from build123d import *

# Parameters (mm, degrees)
SKETCH1_R           = 102.5
BOSS_EXTRUDE1_DEPTH = 41
BOSS_EXTRUDE2_START = 41
SKETCH1_3_R         = 102.5
BOSS_EXTRUDE2_DEPTH = 191
BOSS_EXTRUDE3_START = 232
SKETCH1_4_R         = 102.5
BOSS_EXTRUDE3_DEPTH = 41
SKETCH3_R           = 27.5
SKETCH3_R_2         = 23
SKETCH3_R_3         = 5
BOSS_EXTRUDE4_DEPTH = 10
SKETCH3_3_R         = 23
SKETCH3_3_R_2       = 27.5
BOSS_EXTRUDE5_DEPTH = 273


with BuildPart() as part:
    # Sketch1 → Boss-Extrude1 (new body)
    with BuildSketch(Plane.XY):
        with BuildLine():
            Line((120, 77.892348876), (120, 0))
            Line((120, 0), (80, 0))
            Line((80, 0), (80, 42.168378274))
            ThreePointArc((80, 42.168378274), (0, 19.5), (-80, 42.168378274))
            Line((-80, 42.168378274), (-80, 0))
            Line((-80, 0), (-120, 0))
            Line((-120, 0), (-120, 77.892348876))
            ThreePointArc((-120, 77.892348876), (0, 324.5), (120, 77.892348876))
        make_face()
        with Locations((0, 172)):
            Circle(SKETCH1_R, mode=Mode.SUBTRACT)
        with Locations((0, 172)):
            Circle(SKETCH1_R)
    extrude(amount=BOSS_EXTRUDE1_DEPTH)

    # Sketch1<3> → Boss-Extrude2 (add)
    with BuildSketch(Plane.XY.offset(BOSS_EXTRUDE2_START)):
        with Locations((0, 172)):
            Circle(SKETCH1_3_R)
    extrude(amount=BOSS_EXTRUDE2_DEPTH)

    # Sketch1<4> → Boss-Extrude3 (add)
    with BuildSketch(Plane.XY.offset(BOSS_EXTRUDE3_START)):
        with BuildLine():
            Line((120, 77.892348876), (120, 0))
            Line((120, 0), (80, 0))
            Line((80, 0), (80, 42.168378274))
            ThreePointArc((80, 42.168378274), (0, 19.5), (-80, 42.168378274))
            Line((-80, 42.168378274), (-80, 0))
            Line((-80, 0), (-120, 0))
            Line((-120, 0), (-120, 77.892348876))
            ThreePointArc((-120, 77.892348876), (0, 324.5), (120, 77.892348876))
        make_face()
        with Locations((0, 172)):
            Circle(SKETCH1_4_R, mode=Mode.SUBTRACT)
        with Locations((0, 172)):
            Circle(SKETCH1_4_R)
    extrude(amount=BOSS_EXTRUDE3_DEPTH)

    # Sketch3 → Boss-Extrude4 (add)
    with BuildSketch(Plane.XY):
        Polygon((-273.172788599, 112), (-118.172788599, 112), (-118.172788599, 168.9), (-273.172788599, 168.9), (-343.172788599, 168.9), (-343.172788599, 13.9), (-273.172788599, 13.9), align=None)
        with Locations((-306, 46.9)):
            Circle(SKETCH3_R, mode=Mode.SUBTRACT)
        with Locations((-306, 110.4)):
            Circle(SKETCH3_R_2, mode=Mode.SUBTRACT)
        with Locations((-131, 127)):
            Circle(SKETCH3_R_3, mode=Mode.SUBTRACT)
        with Locations((-131, 156.4)):
            Circle(SKETCH3_R_3, mode=Mode.SUBTRACT)
        with Locations((-306, 46.9)):
            Circle(SKETCH3_R)
        with Locations((-306, 110.4)):
            Circle(SKETCH3_R_2)
    boss_extrude4 = extrude(amount=-BOSS_EXTRUDE4_DEPTH)

    # Mirror1: Boss-Extrude4 across plane
    add(boss_extrude4.mirror(Plane(origin=(0, 0, 136.5), x_dir=(1, 0, 0), z_dir=(0, 0, -1))))

    # Sketch3<3> → Boss-Extrude5 (add)
    with BuildSketch(Plane.XY):
        with Locations((-306, 110.4)):
            Circle(SKETCH3_3_R)
        with Locations((-306, 46.9)):
            Circle(SKETCH3_3_R_2)
    extrude(amount=BOSS_EXTRUDE5_DEPTH)


solid = part.part
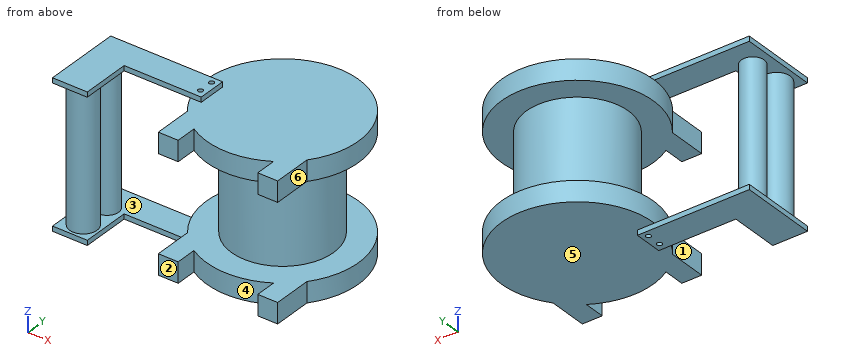
Geometry check sheet. Reference: the model listing, model coordinates, mm. Face numbers are marked on the shaded views. A direction names the side the tool comes from. Round coordinates to 2 decimals unless told otherwise and drop trailing zeros. Write each loop counter-clockwise with the first axis right and the second up, starting at its lowest first coordinate (ties: lowest second). Pieces come first, ordered by that corner, then holes.
Item 1: Section check D-D (y = 186.5). Record the boundary of the cut face in (x, z), plus the area to 3 significant figures.
Determined:
outline: (-151.81, 0) - (151.81, 0) - (151.81, 41) - (101.47, 41) - (101.47, 232) - (151.81, 232) - (151.81, 273) - (-151.81, 273) - (-151.81, 232) - (-101.47, 232) - (-101.47, 41) - (-151.81, 41) - close
area: 63,700 mm2
Item 2: Material ranges on line 1 along Y through (x, z) = (-131, -7); line 2 along Z through (x, y) = (-6, 68); line 3 along Z through (x, y) = (-144, 168), recorded low to high.
Determined:
line 1: y = 112 to 122, 132 to 151.4, 161.4 to 168.9
line 2: z = 0 to 41, 232 to 273
line 3: z = -10 to 41, 232 to 283
Item 3: Section check B-B (x = -257). Record the boundary of the cut face in (y, z).
Determined:
outline: (112, -10) - (168.9, -10) - (168.9, 0) - (112, 0) - close; (112, 273) - (168.9, 273) - (168.9, 283) - (112, 283) - close
Item 4: Go/stop test with flat-tipped pins: pin 1 Ø3 at (y, z) = (71.5, 279.5) entering from +X; pin 2 Ø5 at (y, z) = (132.5, -7) entering from +X; pin 3 Ø20.5 at (y, z) = (51, 261) entering from +X; pin 4 Ø13 at (x, y) = (-131, 156.4) entering from -Z. Record where each tip stops, or that it passes through.
Determined:
pin 1: stops at x = -273.17
pin 2: stops at x = -118.17
pin 3: stops at x = 120
pin 4: stops at z = -10
Item 5: Section check A-A (z = 14). Record the boundary of the cut face in (x, y).
Determined:
outline: circle Ø55 at (-306, 46.9); circle Ø46 at (-306, 110.4); (-120, 0) - (-80, 0) - (-80, 42.17) arc R152.5 ccw to (80, 42.17) - (80, 0) - (120, 0) - (120, 77.89) arc R152.5 ccw (long way) to (-120, 77.89) - close
Item 6: Section check C-C (y = 96). Record the boundary of the cut face in (x, z), plus the area to 3 significant figures.
Determined:
outline: (-343.17, -10) - (-273.17, -10) - (-273.17, 0) - (-288.07, 0) - (-288.07, 273) - (-273.17, 273) - (-273.17, 283) - (-343.17, 283) - (-343.17, 273) - (-323.93, 273) - (-323.93, 0) - (-343.17, 0) - close; (-132.21, 0) - (132.21, 0) - (132.21, 41) - (68.78, 41) - (68.78, 232) - (132.21, 232) - (132.21, 273) - (-132.21, 273) - (-132.21, 232) - (-68.78, 232) - (-68.78, 41) - (-132.21, 41) - close
area: 59,100 mm2
Item 7: Mould release check, pull along X, two halves, no side actions. Record for the marked faces 4, 5 and 6: +X half, -X half, draft (parallel to the pull), parting line (faces both ways), or undercut.
Determined:
face 4: undercut
face 5: draft
face 6: +X half
Item 8: Access from +Z, -Z, +X, -X, +Y, -Y to the whole of each face (thin tool, end or side, straight path). Record for the marked faces 1, 2 and 3.
Determined:
face 1: +Z, -Z, -Y
face 2: +Z, -Z, +X, -X, -Y
face 3: none
